Here's how the part is built. I have some questions about the finished solid (model axes, mm). Round coordinates to 2 decimals unless told otherwise and drop trailing zeros. Loops run counter-clockwise (first coordinate to the right, second up) from the corner with the lowest first, then second, coordinate; pieces in that order, holes last. Notation, with made-up numbers: M -32,58 L -1,58 A28 cw -1,97 Z; hole C 46.5,55.5 d10. An arc over 180 degrees is marked long. Put each result on its own line as item: value. Start each with the question number.
```python
from build123d import *

# Parameters (mm, degrees)
SKETCH1_W                = 51
SKETCH1_H                = 136
BOSS_EXTRUDE1_DEPTH      = 2
CUT_EXTRUDE1_DEPTH       = 10
SKETCH5_W                = 1
SKETCH5_H                = 2
BOSS_EXTRUDE2_DEPTH      = 136
SKETCH6_W                = 1
SKETCH6_H                = 2
BOSS_EXTRUDE3_DEPTH      = 136
SKETCH7_W                = 68.795835126
SKETCH7_H                = 26.425628728
CUT_EXTRUDE2_DEPTH       = 0.4
SKETCH8_W                = 2
SKETCH8_H                = 2
CUT_EXTRUDE3_DEPTH       = 135.6
BOSS_EXTRUDE6_DEPTH      = 10
BOSS_EXTRUDE6_DEPTH_BACK = 10
SKETCH11_R               = 1.5
SKETCH14_R               = 0.62
CUT_EXTRUDE5_DEPTH       = 20


with BuildPart() as part:
    # Sketch1 → Boss-Extrude1 (new body)
    with BuildSketch(Plane(origin=(0, 0, 0), x_dir=(1, 0, 0), z_dir=(0, 1, 0))):
        with Locations((-30.5, -4.545454545)):
            Rectangle(SKETCH1_W, SKETCH1_H)
    extrude(amount=BOSS_EXTRUDE1_DEPTH)

    # Sketch4 → Cut-Extrude1 (cut)
    with BuildSketch(Plane(origin=(0, 2, 0), x_dir=(1, 0, 0), z_dir=(0, 1, 0))):
        with BuildLine():
            Line((-48.1, 58.354545455), (-12.9, 58.354545455))
            ThreePointArc((-12.9, 58.354545455), (-11.9, 57.354545455), (-12.9, 56.354545455))
            Line((-12.9, 56.354545455), (-48.1, 56.354545455))
            ThreePointArc((-48.1, 56.354545455), (-49.1, 57.354545455), (-48.1, 58.354545455))
        make_face()
        with BuildLine():
            Line((-48.1, 54.354545455), (-12.9, 54.354545455))
            ThreePointArc((-12.9, 54.354545455), (-11.9, 53.354545455), (-12.9, 52.354545455))
            Line((-12.9, 52.354545455), (-48.1, 52.354545455))
            ThreePointArc((-48.1, 52.354545455), (-49.1, 53.354545455), (-48.1, 54.354545455))
        make_face()
        with BuildLine():
            Line((-48.1, 50.354545455), (-12.9, 50.354545455))
            ThreePointArc((-12.9, 50.354545455), (-11.9, 49.354545455), (-12.9, 48.354545455))
            Line((-12.9, 48.354545455), (-48.1, 48.354545455))
            ThreePointArc((-48.1, 48.354545455), (-49.1, 49.354545455), (-48.1, 50.354545455))
        make_face()
        with BuildLine():
            Line((-48.1, 46.354545455), (-12.9, 46.354545455))
            ThreePointArc((-12.9, 46.354545455), (-11.9, 45.354545455), (-12.9, 44.354545455))
            Line((-12.9, 44.354545455), (-48.1, 44.354545455))
            ThreePointArc((-48.1, 44.354545455), (-49.1, 45.354545455), (-48.1, 46.354545455))
        make_face()
        with BuildLine():
            Line((-48.1, 42.354545455), (-12.9, 42.354545455))
            ThreePointArc((-12.9, 42.354545455), (-11.9, 41.354545455), (-12.9, 40.354545455))
            Line((-12.9, 40.354545455), (-48.1, 40.354545455))
            ThreePointArc((-48.1, 40.354545455), (-49.1, 41.354545455), (-48.1, 42.354545455))
        make_face()
        with BuildLine():
            Line((-48.1, 38.354545455), (-12.9, 38.354545455))
            ThreePointArc((-12.9, 38.354545455), (-11.9, 37.354545455), (-12.9, 36.354545455))
            Line((-12.9, 36.354545455), (-48.1, 36.354545455))
            ThreePointArc((-48.1, 36.354545455), (-49.1, 37.354545455), (-48.1, 38.354545455))
        make_face()
        with BuildLine():
            Line((-48.1, 34.354545455), (-12.9, 34.354545455))
            ThreePointArc((-12.9, 34.354545455), (-11.9, 33.354545455), (-12.9, 32.354545455))
            Line((-12.9, 32.354545455), (-48.1, 32.354545455))
            ThreePointArc((-48.1, 32.354545455), (-49.1, 33.354545455), (-48.1, 34.354545455))
        make_face()
        with BuildLine():
            Line((-48.1, 30.354545455), (-12.9, 30.354545455))
            ThreePointArc((-12.9, 30.354545455), (-11.9, 29.354545455), (-12.9, 28.354545455))
            Line((-12.9, 28.354545455), (-48.1, 28.354545455))
            ThreePointArc((-48.1, 28.354545455), (-49.1, 29.354545455), (-48.1, 30.354545455))
        make_face()
        with BuildLine():
            Line((-48.1, 26.354545455), (-12.9, 26.354545455))
            ThreePointArc((-12.9, 26.354545455), (-11.9, 25.354545455), (-12.9, 24.354545455))
            Line((-12.9, 24.354545455), (-48.1, 24.354545455))
            ThreePointArc((-48.1, 24.354545455), (-49.1, 25.354545455), (-48.1, 26.354545455))
        make_face()
        with BuildLine():
            Line((-48.1, 22.354545455), (-12.9, 22.354545455))
            ThreePointArc((-12.9, 22.354545455), (-11.9, 21.354545455), (-12.9, 20.354545455))
            Line((-12.9, 20.354545455), (-48.1, 20.354545455))
            ThreePointArc((-48.1, 20.354545455), (-49.1, 21.354545455), (-48.1, 22.354545455))
        make_face()
        with BuildLine():
            Line((-48.1, 18.354545455), (-12.9, 18.354545455))
            ThreePointArc((-12.9, 18.354545455), (-11.9, 17.354545455), (-12.9, 16.354545455))
            Line((-12.9, 16.354545455), (-48.1, 16.354545455))
            ThreePointArc((-48.1, 16.354545455), (-49.1, 17.354545455), (-48.1, 18.354545455))
        make_face()
        with BuildLine():
            Line((-48.1, 14.354545455), (-12.9, 14.354545455))
            ThreePointArc((-12.9, 14.354545455), (-11.9, 13.354545455), (-12.9, 12.354545455))
            Line((-12.9, 12.354545455), (-48.1, 12.354545455))
            ThreePointArc((-48.1, 12.354545455), (-49.1, 13.354545455), (-48.1, 14.354545455))
        make_face()
        with BuildLine():
            Line((-48.1, 10.354545455), (-12.9, 10.354545455))
            ThreePointArc((-12.9, 10.354545455), (-11.9, 9.354545455), (-12.9, 8.354545455))
            Line((-12.9, 8.354545455), (-48.1, 8.354545455))
            ThreePointArc((-48.1, 8.354545455), (-49.1, 9.354545455), (-48.1, 10.354545455))
        make_face()
    extrude(amount=-CUT_EXTRUDE1_DEPTH, mode=Mode.SUBTRACT)

    # Sketch5 → Boss-Extrude2 (add)
    with BuildSketch(Plane(origin=(0, 0, -63.454545455), x_dir=(-1, 0, 0), z_dir=(0, 0, -1))):
        with Locations((56.5, 1)):
            Rectangle(SKETCH5_W, SKETCH5_H)
        with Locations((4.5, 1)):
            Rectangle(SKETCH5_W, SKETCH5_H)
    extrude(amount=-BOSS_EXTRUDE2_DEPTH)

    # Sketch6 → Boss-Extrude3 (add)
    with BuildSketch(Plane(origin=(0, 0, -63.454545455), x_dir=(-1, 0, 0), z_dir=(0, 0, -1))):
        with Locations((57.5, 1)):
            Rectangle(SKETCH6_W, SKETCH6_H)
        with Locations((3.5, 1)):
            Rectangle(SKETCH6_W, SKETCH6_H)
    extrude(amount=-BOSS_EXTRUDE3_DEPTH)

    # Sketch7 → Cut-Extrude2 (cut)
    with BuildSketch(Plane.XY.offset(72.545454545)):
        with Locations((-32.339758962, -3.400766566)):
            Rectangle(SKETCH7_W, SKETCH7_H)
    extrude(amount=-CUT_EXTRUDE2_DEPTH, mode=Mode.SUBTRACT)

    # Sketch8 → Cut-Extrude3 (cut)
    with BuildSketch(Plane(origin=(0, 0, -63.454545455), x_dir=(-1, 0, 0), z_dir=(0, 0, -1))):
        with Locations((4, 1)):
            Rectangle(SKETCH8_W, SKETCH8_H)
        with Locations((57, 1)):
            Rectangle(SKETCH8_W, SKETCH8_H)
    extrude(amount=-CUT_EXTRUDE3_DEPTH, mode=Mode.SUBTRACT)

    # Sketch11 → Boss-Extrude6 (add, two sides: drawn at the far end of the back side and taken through both)
    with BuildSketch(Plane.ZY.offset(30.5).offset(-BOSS_EXTRUDE6_DEPTH_BACK)):
        with Locations((72.145454545, 2.5)):
            Circle(SKETCH11_R)
    extrude(amount=BOSS_EXTRUDE6_DEPTH + BOSS_EXTRUDE6_DEPTH_BACK)

    # Sketch14 → Cut-Extrude5 (cut)
    with BuildSketch(Plane.ZY.offset(40.5)):
        with Locations(Location((72.145454545, 3, 0), (0, 0, 270))):
            Circle(SKETCH14_R)
    extrude(amount=-CUT_EXTRUDE5_DEPTH, mode=Mode.SUBTRACT)


solid = part.part
```
1) If I drill on probe 1 along Y at (x, z) = (-53, -56); probe 2 along Z at (x, y) = (-29, 3); probe 3 along Z at (x, y) = (-50.5, 1.9), over which ranges is the centre line in solid material (lowest first)? Write a range as from..to.
2) Suppose I cut it at A-A (y = 3). Write out the boundary of the cut face in (x, z), plus the area to 3 significant figures.
3) Suppose I cut it at B-B (x = -34). State how many separate pieces and enclosed holes the cut face has, plus the area to 3 significant figures.
4) Suppose I cut it at C-C (z = 21.5). Write out the boundary of the cut face in (x, y).
5) I'm going to push flat-ended pins straight in: P1, Ø1.6, axis at x = -18, y = 1.5, coming from the +Z side; P2, Ø2, axis at x = -37.5, y = 1, coming from the +Z side; P3, Ø1.6, axis at x = -26, y = 1, coming from the +Z side. Where does each tip first touch, or does it pass through?
Results are:
1. probe 1: 0..2
1. probe 2: 70.73..71.53, 72.77..73.56
1. probe 3: -63.45..72.15
2. outline: M -40.5,70.73 L -20.5,70.73 L -20.5,71.53 L -40.5,71.53 Z; M -40.5,72.77 L -20.5,72.77 L -20.5,73.56 L -40.5,73.56 Z
2. area: 31.8 mm²
3. separate pieces: 14
3. enclosed holes: 1
3. area: 224 mm²
4. outline: M -56,0 L -5,0 L -5,2 L -56,2 Z
5. P1: z = 72.15
5. P2: z = 73.56
5. P3: z = 73.47
